Work out the finished part from the listing and answer in its coordinate system (mm). Face numbers are marked on the shaded views. A direction names the side the tool comes from. Round coordinates to 2 decimals unless told otherwise and drop trailing zeros. Write each loop counter-clockwise with the first axis right and the second up, starting at its lowest first coordinate (ties: lowest second). Pieces come first, ordered by that corner, then holes. Notation, with made-up numbers: M 69,53 L 126,53 A34 ccw 126,91 Z; hole C 24,-20 d6. An arc over 180 degrees is marked long. Answer in a Markdown table with one row per item.
```python
from build123d import *

# Parameters (mm, degrees)
SKETCH1_R             = 25
BOSS_EXTRUDE1_DEPTH   = 4
SKETCH2_R             = 10
BOSS_EXTRUDE2_DEPTH   = 7
FILLET1_R             = 1
SKETCH3_R             = 7.5
CUT_EXTRUDE1_DEPTH    = 5
F_6_0MM_DOWEL_HOLE1_D = 6.8


with BuildPart() as part:
    # Sketch1 → Boss-Extrude1 (new body)
    with BuildSketch(Plane.XY):
        Circle(SKETCH1_R)
    extrude(amount=-BOSS_EXTRUDE1_DEPTH)

    # Sketch2 → Boss-Extrude2 (add)
    with BuildSketch(Plane.XY):
        Circle(SKETCH2_R)
    extrude(amount=BOSS_EXTRUDE2_DEPTH)

    # Fillet1
    fillet1_edges = [part.edges().sort_by_distance(p)[0] for p in [
        (-10, 0, 0),
    ]]
    fillet(fillet1_edges, radius=FILLET1_R)

    # Sketch3 → Cut-Extrude1 (cut)
    with BuildSketch(Plane(origin=(0, 0, -4), x_dir=(-1, 0, 0), z_dir=(0, 0, -1))):
        Circle(SKETCH3_R)
    extrude(amount=-CUT_EXTRUDE1_DEPTH, mode=Mode.SUBTRACT)

    # Ø6.0mm Dowel Hole1 (through all)
    with Locations(Plane.XY):
        with Locations((-12.990381057, -7.5), (0, 15), (12.990381057, -7.5)):
            Hole(F_6_0MM_DOWEL_HOLE1_D / 2)


solid = part.part
```
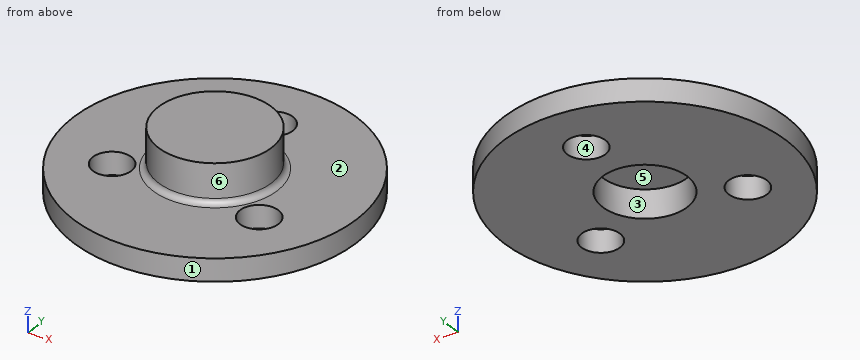
1. Consider line 1 along Y through (x, z) = (0, -1.8); line 2 along X through (y, z) = (-9, -0.75); line 3 along Z through (x, y) = (0.5, -14.5). Determine where each line is inside the solid, lowest interval first. Write a range as from..to.
Calculated:
| item | result |
|---|---|
| line 1 | y = -25..-7.5, 7.5..11.6, 18.4..25 |
| line 2 | x = -23.32..-16.04, -9.94..9.94, 16.04..23.32 |
| line 3 | z = -4..0 |
2. The part is cut by section A-A (x = 0). Determine the outline of the cut face in (y, z).
Calculated:
| item | result |
|---|---|
| outline | M -25,-4 L -7.5,-4 L -7.5,1 L 7.5,1 L 7.5,-4 L 11.6,-4 L 11.6,0 L 11,0 A1 cw 10,1 L 10,7 L -10,7 L -10,1 A1 cw -11,0 L -25,0 Z; M 18.4,-4 L 25,-4 L 25,0 L 18.4,0 Z |
3. Determine the mould class of the marked faces 1, 2 and 3 for opening direction Y: released by +Y, released by -Y, zero draft, split by the parting line, or undercut.
Calculated:
| item | result |
|---|---|
| face 1 | split by the parting line |
| face 2 | zero draft |
| face 3 | undercut |
4. The part is cut by section D-D (y = 0). Determine the outline of the cut face in (x, z), plus the area to 3 significant figures.
Calculated:
| item | result |
|---|---|
| outline | M -25,-4 L -7.5,-4 L -7.5,1 L 7.5,1 L 7.5,-4 L 25,-4 L 25,0 L 11,0 A1 cw 10,1 L 10,7 L -10,7 L -10,1 A1 cw -11,0 L -25,0 Z |
| area | 265 mm² |
5. The part is cut by section C-C (z = -0.75). Determine the outline of the cut face in (x, y).
Calculated:
| item | result |
|---|---|
| outline | C 0,0 d50; hole C -12.99,-7.5 d6.8; hole C 0,0 d15; hole C 0,15 d6.8; hole C 12.99,-7.5 d6.8 |
6. A tool of negligible diameter and unlimited length cuts with its end or side. For the marked faces 4, 5 and 6, from which of +Z, -Z, +X, -X, +Y, -Y can it reach the whole face along a straight path? Write none if from no direction.
Calculated:
| item | result |
|---|---|
| face 4 | +Z, -Z |
| face 5 | -Z |
| face 6 | +Z |
7. The part is cut by section B-B (y = 15). Determine the outline of the cut face in (x, z).
Calculated:
| item | result |
|---|---|
| outline | M -20,-4 L -3.4,-4 L -3.4,0 L -20,0 Z; M 3.4,-4 L 20,-4 L 20,0 L 3.4,0 Z |
8. Given pin 1 (1.5 mm diameter, centred on x = -7, z = 5, fed in from -Y); pin 2 (1.5 mm diameter, centred on y = 19, z = 0, fed in from -X); pin 3 (6 mm diameter, centred on x = 12.99, y = -7.5, fed in from -Z), each flat-ended and moving along its own axis, determine where each tip first touches the part or whether it passes through.
Calculated:
| item | result |
|---|---|
| pin 1 | stops at y = -7.81 |
| pin 2 | stops at x = -17.09 |
| pin 3 | passes through |
